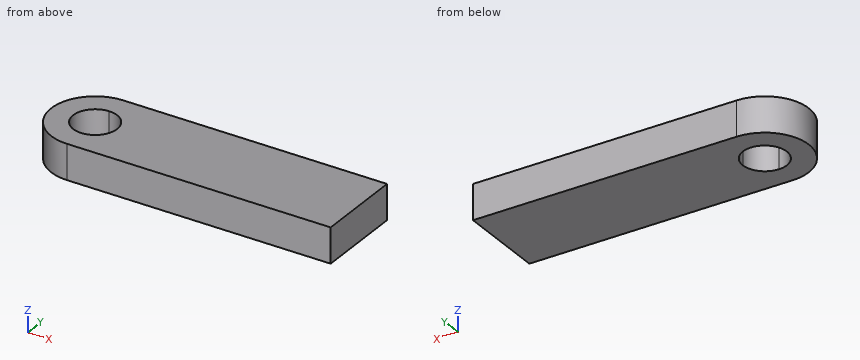
```python
from build123d import *

# Parameters (mm, degrees)
F1_DEPTH = 20


with BuildPart() as f1:
    # F0 (on Top) → F1 (new body)
    with BuildSketch(Plane.XY):
        with BuildLine():
            ThreePointArc((-50, 0), (-57.3223304703, 17.6776695297), (-75, 25))
            Line((-75, 25), (-75, 12.5))
            ThreePointArc((-75, 12.5), (-66.1611652352, 8.8388347648), (-62.5, 0))
            ThreePointArc((-62.5, 0), (-66.1611652352, -8.8388347648), (-75, -12.5))
            Line((-75, -12.5), (-75, -25))
            ThreePointArc((-75, -25), (-57.3223304703, -17.6776695297), (-50, 0))
        make_face()
        with BuildLine():
            Line((75, 25), (-75, 25))
            ThreePointArc((-75, 25), (-57.3223304703, 17.6776695297), (-50, 0))
            ThreePointArc((-50, 0), (-57.3223304703, -17.6776695297), (-75, -25))
            Line((-75, -25), (75, -25))
            Line((75, -25), (75, 25))
        make_face()
        with BuildLine():
            Line((-75, 12.5), (-75, 25))
            ThreePointArc((-75, 25), (-100, 0), (-75, -25))
            Line((-75, -25), (-75, -12.5))
            ThreePointArc((-75, -12.5), (-87.5, 0), (-75, 12.5))
        make_face()
    extrude(amount=F1_DEPTH)


solid = f1.part
```
Input: part model. Units: mm. Frame: model coordinates. Give positions to 0.01 mm unless a question says otherwise; leave off trailing zeros. Order: outer loops, then holes, each group sorted by start corner. A loop starts at its lowest first (then second) coordinate and runs counter-clockwise, first axis right, second up.
1. Section B-B on y = -6.5. Return the cut outline in (x, z), and give its area (3 significant figures).
Derived:
outline: (-99.14, 0) - (-85.68, 0) - (-85.68, 20) - (-99.14, 20) - close; (-64.32, 0) - (75, 0) - (75, 20) - (-64.32, 20) - close
area: 3,060 mm2
2. Section D-D on y = -22. Return the cut outline in (x, z), and give its area (3 significant figures).
Derived:
outline: (-86.87, 0) - (75, 0) - (75, 20) - (-86.87, 20) - close
area: 3,240 mm2
3. Section C-C on y = 2.5. Return the cut outline in (x, z).
Derived:
outline: (-99.87, 0) - (-87.25, 0) - (-87.25, 20) - (-99.87, 20) - close; (-62.75, 0) - (75, 0) - (75, 20) - (-62.75, 20) - close
4. Material intervals for L1, parallel to X at y = 11, z = 7.75; L2, parallel to X at y = -11.5, z = 17.5; L3, parallel to Y at x = -67.5, z = 4.25, sorted ascending.
Derived:
L1: x = -97.45 to -80.94, -69.06 to 75
L2: x = -97.2 to -79.9, -70.1 to 75
L3: y = -25 to -10, 10 to 25
5. Section A-A on z = 3.25. Return the cut outline in (x, y), and give its area (3 significant figures).
Derived:
outline: (-75, -25) - (75, -25) - (75, 25) - (-75, 25) arc R25 ccw to start; hole circle Ø25 at (-75, 0)
area: 7,990 mm2
6. Pin query (flat end, axial travel): pin 1 (12 mm diameter, centred on y = 19, z = 10, fed in from -X); pin 2 (5 mm diameter, centred on y = 4.5, z = 6.5, fed in from -X). Return the tip coordinate at first contact, or that it passes through.
Derived:
pin 1: stops at x = -96.35
pin 2: stops at x = -99.92
